The model under review builds one solid part; all positions refer to its coordinate system, in mm. A direction names the side the tool comes from. Round coordinates to 2 decimals unless told otherwise and drop trailing zeros. Write each loop counter-clockwise with the first axis right and the second up, starting at its lowest first coordinate (ties: lowest second). Pieces come first, ordered by that corner, then holes. Notation, with made-up numbers: (-24.75, 73.25) -> (34.25, 73.25) arc R6 cw to (34.25, 83.25) -> close; hole circle Ø4 at (-8.5, 30). An arc over 180 degrees is marked (long way). Use CSV: the item, a comma, the result in double quotes. Start each with the question number.
1) Wall thickness on probe 1 along X at (y, z) = (0.4, 10); probe 2 along X at (y, z) = (0.25, 5); probe 3 along Z at (x, y) = (-48.25, 0.7): over which ranges is each line inside the solid? List them lowest first. Write a range as [from, to].
2) Machinability: for faces 1 (the face through (-37.483, 0.5, 19.5)), 2 (the face through (-48.8, 0.5, 18.055)), 3 (the face through (-22.9, 0.5, 18.78)), which of the approach directions +Z, -Z, +X, -X, +Y, -Y give a long, thin tool a straight path to every point of the face, cutting with its end or side? Answer none if there is none.
3) Take a section at A-A, the plane x = -48.25. Give the boundary of the cut face in (y, z), then the cut area to 3 significant figures.
4) Take a section at C-C, the plane y = 0.2. Give the boundary of the cut face in (x, z).
5) Mouldability with a two-part tool opening along X and no side actions: class faces 4 (the face through (-38.9, 0.5, 20.28)), 5 (the face through (-40.233, 0.5, 4.6)), 6 (the face through (-32.4, 0.5, 18.78)) as released by +X, released by -X, zero draft, split by the parting line, or undercut.
6) For pin 1 Ø0.5 at (x, y) = (-49, 0.5) entering from -Z; pin 2 Ø0.5 at (x, y) = (-32, 0.5) entering from +Z, all flat-tipped, find the tip position at first contact; note any pin that passes through.
7) Take a section at B-B, the plane z = 6.75. Give the boundary of the cut face in (x, y).
from build123d import *

# Parameters (mm, degrees)
SKETCH1_W              = 29.5
SKETCH1_H              = 13.45
BOSS_EXTRUDE1_DEPTH    = 1
SKETCH2_W              = 2.75
SKETCH2_H              = 1.5
BOSS_EXTRUDE2_DEPTH    = 1
SKETCH3_W              = 2.12
SKETCH3_H              = 12
ADAPTER_PCB_HOLE_DEPTH = 1


with BuildPart() as part:
    # Sketch1 → Boss-Extrude1 (new body)
    with BuildSketch(Plane(origin=(0, 0, 0), x_dir=(1, 0, 0), z_dir=(0, 1, 0))):
        with Locations((-36.048423651, -12.055454233)):
            Rectangle(SKETCH1_W, SKETCH1_H)
    extrude(amount=BOSS_EXTRUDE1_DEPTH)

    # Sketch2 → Boss-Extrude2 (add)
    with BuildSketch(Plane(origin=(0, 0, 0), x_dir=(1, 0, 0), z_dir=(0, 1, 0))):
        with Locations((-38.858423651, -4.580454233)):
            Rectangle(SKETCH2_W, SKETCH2_H)
        with Locations((-38.858423651, -19.530454233)):
            Rectangle(SKETCH2_W, SKETCH2_H)
        with Locations((-25.858423651, -4.580454233)):
            Rectangle(SKETCH2_W, SKETCH2_H)
        with Locations((-25.858423651, -19.530454233)):
            Rectangle(SKETCH2_W, SKETCH2_H)
    extrude(amount=BOSS_EXTRUDE2_DEPTH)

    # Sketch3 → adapter_PCB_hole (cut)
    with BuildSketch(Plane(origin=(0, 0, 0), x_dir=(-1, 0, 0), z_dir=(0, -1, 0))):
        with Locations((48.858423651, -12.055454233)):
            Rectangle(SKETCH3_W, SKETCH3_H)
    extrude(amount=-ADAPTER_PCB_HOLE_DEPTH, mode=Mode.SUBTRACT)


solid = part.part
Values found:
1,probe 1,"[-50.8, -49.92], [-47.8, -21.3]"
1,probe 2,"[-40.23, -37.48], [-27.23, -24.48]"
1,probe 3,"[5.33, 6.06], [18.06, 18.78]"
2,face 1,"+Z, +Y, -Y"
2,face 2,"+Y, -Y"
2,face 3,"+Z, +X, +Y, -Y"
3,outline,"(0, 5.33) -> (1, 5.33) -> (1, 6.06) -> (0, 6.06) -> close; (0, 18.06) -> (1, 18.06) -> (1, 18.78) -> (0, 18.78) -> close"
3,area,"1.45 mm²"
4,outline,"(-50.8, 5.33) -> (-40.23, 5.33) -> (-40.23, 3.83) -> (-37.48, 3.83) -> (-37.48, 5.33) -> (-27.23, 5.33) -> (-27.23, 3.83) -> (-24.48, 3.83) -> (-24.48, 5.33) -> (-21.3, 5.33) -> (-21.3, 18.78) -> (-24.48, 18.78) -> (-24.48, 20.28) -> (-27.23, 20.28) -> (-27.23, 18.78) -> (-37.48, 18.78) -> (-37.48, 20.28) -> (-40.23, 20.28) -> (-40.23, 18.78) -> (-50.8, 18.78) -> close; hole (-49.92, 6.06) -> (-47.8, 6.06) -> (-47.8, 18.06) -> (-49.92, 18.06) -> close"
5,face 4,"zero draft"
5,face 5,"released by -X"
5,face 6,"undercut"
6,pin 1,"z = 5.33"
6,pin 2,"z = 18.78"
7,outline,"(-50.8, 0) -> (-49.92, 0) -> (-49.92, 1) -> (-50.8, 1) -> close; (-47.8, 0) -> (-21.3, 0) -> (-21.3, 1) -> (-47.8, 1) -> close"
